from build123d import *

# Parameters (mm, degrees)
SCHIZZO2_R                   = 23
SCHIZZO2_R_2                 = 2.8
ESTRUSIONE_ESTRUSIONE3_DEPTH = 5
SCHIZZO5_R                   = 4.3
TAGLIO_ESTRUSIONE1_DEPTH     = 3
SCHIZZO6_R                   = 9.8
TAGLIO_ESTRUSIONE2_DEPTH     = 33.908965344


with BuildPart() as part:
    # Schizzo2 → Estrusione-Estrusione3 (new body)
    with BuildSketch(Plane.XY):
        Circle(SCHIZZO2_R)
        with Locations((-12.727922061, 12.727922061)):
            Circle(SCHIZZO2_R_2, mode=Mode.SUBTRACT)
        with Locations((12.727922061, 12.727922061)):
            Circle(SCHIZZO2_R_2, mode=Mode.SUBTRACT)
        with Locations((12.727922061, -12.727922061)):
            Circle(SCHIZZO2_R_2, mode=Mode.SUBTRACT)
        with Locations((-12.727922061, -12.727922061)):
            Circle(SCHIZZO2_R_2, mode=Mode.SUBTRACT)
    extrude(amount=ESTRUSIONE_ESTRUSIONE3_DEPTH)

    # Schizzo5 → Taglio-Estrusione1 (cut)
    with BuildSketch(Plane(origin=(0, 0, 0), x_dir=(-1, 0, 0), z_dir=(0, 0, -1))):
        with Locations((-12.727922061, 12.727922061)):
            Circle(SCHIZZO5_R)
        with Locations((12.758824691, 12.727922061)):
            Circle(SCHIZZO5_R)
        with Locations((12.727922061, -12.727922061)):
            Circle(SCHIZZO5_R)
        with Locations((-12.727922061, -12.727922061)):
            Circle(SCHIZZO5_R)
    extrude(amount=-TAGLIO_ESTRUSIONE1_DEPTH, mode=Mode.SUBTRACT)

    # Schizzo6 → Taglio-Estrusione2 (cut, through all)
    with BuildSketch(Plane(origin=(0, 0, 0), x_dir=(-1, 0, 0), z_dir=(0, 0, -1))):
        Circle(SCHIZZO6_R)
    extrude(amount=-TAGLIO_ESTRUSIONE2_DEPTH, mode=Mode.SUBTRACT)


solid = part.part
Build history of the part. All positions in model axes, mm. A direction names the side the tool comes from. Coordinates: 2 decimals unless noted, no trailing zeros. Write each loop counter-clockwise with the first axis right and the second up, starting at its lowest first coordinate (ties: lowest second). Pieces come first, ordered by that corner, then holes.
(1) Cut at C-C on z = 4.25. List the corners of the cut face in (x, y).
(2) Pin check, flat tips, straight feed: pin 1 Ø7.5 at (x, y) = (12.73, 12.73) entering from -Z; pin 2 Ø4.5 at (x, y) = (-12.73, 12.73) entering from +Z; pin 3 Ø1.5 at (y, z) = (4.5, 3.5) entering from +X; pin 4 Ø1 at (x, z) = (-3.5, 4.5) entering from -Y. Stop position of each tip, or through.
(3) Cut at D-D on x = -20. List the corners of the cut face in (y, z).
(4) 3-axis set-ups, long thin cutter, end or side, ignore diameter. For faces 4 (the flat face through (-16, 13, 3)), 5 (the cylindrical face through (12.1, 10, 4)): which of +Z, -Z, +X, -X, +Y, -Y reach the whole face in a straight line?
(5) Mould opens along Y. For faces 1 (the cylindrical face through (-10.057, -11.887, 3.986)), 2 (the flat face through (10, 0, 5)), 3 (the cylindrical face through (-2.994, 22.804, 2.465)) say: pulls with the +Y half, pulls with the -Y half, needs draft (parallel to the pull), parting line crosses it, or undercut.
(6) Drill centre lines: line 1 (X direction, y = 14, z = 0.85); line 2 (Y direction, x = -11, z = 1.4); line 3 (X direction, y = 12, z = 0.85). Where is each one in solid material? Low to high.
(7) Cut at A-A on y = 0. List the corners of the cut face in (x, z).
Working result:
1. outline: circle Ø46 at (0, 0); hole circle Ø5.6 at (-12.73, -12.73); hole circle Ø5.6 at (-12.73, 12.73); hole circle Ø19.6 at (0, 0); hole circle Ø5.6 at (12.73, -12.73); hole circle Ø5.6 at (12.73, 12.73)
2. pin 1: stops at z = 3
2. pin 2: passes through
2. pin 3: stops at x = 22.69
2. pin 4: stops at y = -22.8
3. outline: (-11.36, 0) - (11.36, 0) - (11.36, 5) - (-11.36, 5) - close
4. face 4: -Z
4. face 5: +Z, -Z
5. face 1: undercut
5. face 2: needs draft
5. face 3: parting line crosses it
6. line 1: x = -18.25 to -16.87, -8.65 to 8.62, 16.84 to 18.25
6. line 2: y = -20.2 to -16.67, -8.79 to 8.8, 16.65 to 20.2
6. line 3: x = -19.62 to -17, -8.52 to 8.49, 16.97 to 19.62
7. outline: (-23, 0) - (-9.8, 0) - (-9.8, 5) - (-23, 5) - close; (9.8, 0) - (23, 0) - (23, 5) - (9.8, 5) - close
